CAD build for the part. Positions are in the model's coordinates, mm. A direction names the side the tool comes from. Round coordinates to 2 decimals unless told otherwise and drop trailing zeros. Write each loop counter-clockwise with the first axis right and the second up, starting at its lowest first coordinate (ties: lowest second). Pieces come first, ordered by that corner, then holes. Notation, with made-up numbers: (2, 3) -> (25, 3) arc R36 ccw to (25, 42) -> close; hole circle Ø3 at (-37, -6). An arc over 180 degrees is marked (long way). Put each result on its own line as item: value. Start each with the question number.
1. Saw through at A-A on y = -0.75. List the corners of the cut face in (x, z), and give its area (3 significant figures).
2. Saw through at B-B on z = 12.25. State how many separate pieces and enclosed holes the cut face has, and give its area (3 significant figures).
3. Saw through at C-C on x = 3.25. List the corners of the cut face in (y, z).
4. 3-axis set-ups, long thin cutter, end or side, ignore diameter. For faces 5 (the flat face through (6, 1, 7.4)), 6 (the flat face through (6, 1, 11.4)), 7 (the flat face through (5.3, -1, 8)): which of +Z, -Z, +X, -X, +Y, -Y reach the whole face in a straight line?
5. Drill centre lines: line 1 (Z direction, x = 8.3, y = 3.1); line 2 (Z direction, x = 7.25, y = 5.5); line 3 (X direction, y = -0.75, z = 15.25). Where is each one in solid material? Low to high. Write a range as from..to.
6. Pull direction Y, two halves, no side cores. Call faces 1 (the cylindrical face through (-0.27, -1.22, 8.48)), 2 (the cylindrical face through (10, 3.34, 3.53)), 3 (the cylindrical face through (-2.7, 0.1, 8.5)), 4 (the flat face through (3, -2.7, 8)): pulls with the +Y half, pulls with the -Y half, needs draft (parallel to the pull), parting line crosses it, or undercut.
7. Flat gauge pins, fed straight in: P1, Ø1.4, axis at x = 6.5, y = 0.5, coming from the +Z side; P2, Ø1.5, axis at y = 2.5, z = 12.5, coming from the -X side; P3, Ø1.5, axis at y = -1.5, z = 12, coming from the +X side; P4, Ø1, axis at x = 3, y = 3, coming from the -Z side. Where does each tip first touch, or does it go through?
8. Saw through at D-D on y = -2. List the corners of the cut face in (x, z).
from build123d import *

# Parameters (mm, degrees)
SKETCH_1_R                = 1.25
EXTRUDE_1_DEPTH           = 17.2
CUT_EXTRUDE_1_DEPTH       = 9.6
HOLE_WIZARD_1_D           = 3.4
HOLE_WIZARD_1_DEPTH       = 3.5
HOLE_WIZARD_1_CSINK_D     = 6.6
HOLE_WIZARD_1_CSINK_ANGLE = 90
HOLE_WIZARD_1_TIP         = 1.021463052
EXTRUDE_3_DEPTH           = 4


with BuildPart() as part:
    # 草图1 → 凸台-拉伸1 (new body)
    with BuildSketch(Plane.XY):
        with BuildLine():
            Line((0, -2.7), (5.3, -2.7))
            Line((5.3, -2.7), (5.3, 2.3))
            Line((5.3, 2.3), (12.8, 2.3))
            Line((12.8, 2.3), (12.8, 5.9))
            Line((12.8, 5.9), (4.3, 5.9))
            ThreePointArc((4.3, 5.9), (2.680018657, 3.58778743), (0, 2.7))
            ThreePointArc((0, 2.7), (-2.7, 0), (0, -2.7))
        make_face()
        Circle(SKETCH_1_R, mode=Mode.SUBTRACT)
    extrude(amount=EXTRUDE_1_DEPTH)

    # 草图2 → 切除-拉伸1 (cut, through all)
    with BuildSketch(Plane(origin=(0, 5.9, 0), x_dir=(1, 0, 0), z_dir=(0, 1, 0))):
        with BuildLine():
            Line((12.8, -17.2), (12.8, 0))
            Line((12.8, 0), (8.3, 0))
            ThreePointArc((8.3, 0), (10.845584412, -1.054415588), (11.9, -3.6))
            ThreePointArc((11.9, -3.6), (11.874356619, -4.028922794), (11.797791798, -4.451735016))
            ThreePointArc((11.797791798, -4.451735016), (11.3, -8.6), (11.797791798, -12.748264984))
            ThreePointArc((11.797791798, -12.748264984), (11.874356619, -13.171077206), (11.9, -13.6))
            ThreePointArc((11.9, -13.6), (10.845584412, -16.145584412), (8.3, -17.2))
            Line((8.3, -17.2), (12.8, -17.2))
        make_face()
    extrude(amount=-CUT_EXTRUDE_1_DEPTH, mode=Mode.SUBTRACT)

    # 打孔尺寸(%根据)开槽半沉头木螺钉的类型1
    with Locations(Plane(origin=(8.3, 5.9, 3.6), x_dir=(1, 0, 0), z_dir=(0, 1, 0))):
        with Locations((0, 0), (0, -10)):
            CounterSinkHole(HOLE_WIZARD_1_D / 2, HOLE_WIZARD_1_CSINK_D / 2, depth=HOLE_WIZARD_1_DEPTH, counter_sink_angle=HOLE_WIZARD_1_CSINK_ANGLE)
            with Locations((0, 0, -(HOLE_WIZARD_1_DEPTH + HOLE_WIZARD_1_TIP / 2))):  # 118° drill point
                Cone(0, HOLE_WIZARD_1_D / 2, HOLE_WIZARD_1_TIP, mode=Mode.SUBTRACT)

    # 草图5 → 凸台-拉伸3 (add)
    with BuildSketch(Plane.XY.offset(7.4)):
        Polygon((5.3, 2.3), (5.3, -0.528427125), (8.128427125, 2.3), align=None)
    extrude(amount=EXTRUDE_3_DEPTH)


solid = part.part
Return value:
1. outline: (-2.59, 0) -> (-1, 0) -> (-1, 17.2) -> (-2.59, 17.2) -> close; (1, 0) -> (5.3, 0) -> (5.3, 17.2) -> (1, 17.2) -> close
1. area: 101 mm^2
2. separate pieces: 2
2. enclosed holes: 1
2. area: 54.2 mm^2
3. outline: (-2.7, 0) -> (4.09, 0) -> (4.09, 17.2) -> (-2.7, 17.2) -> close
4. face 5: -Z, +X, -Y
4. face 6: +Z, +X, -Y
4. face 7: +X, -Y
5. line 1: z = 0..1.9, 5.3..11.9, 15.3..17.2
5. line 2: z = 0..0.9, 6.3..10.9, 16.3..17.2
5. line 3: x = -2.59..-1, 1..5.3
6. face 1: undercut
6. face 2: needs draft
6. face 3: parting line crosses it
6. face 4: pulls with the -Y half
7. P1: stops at z = 11.4
7. P2: stops at x = -2.06
7. P3: stops at x = 5.3
7. P4: stops at z = 0
8. outline: (-1.81, 0) -> (5.3, 0) -> (5.3, 17.2) -> (-1.81, 17.2) -> close
